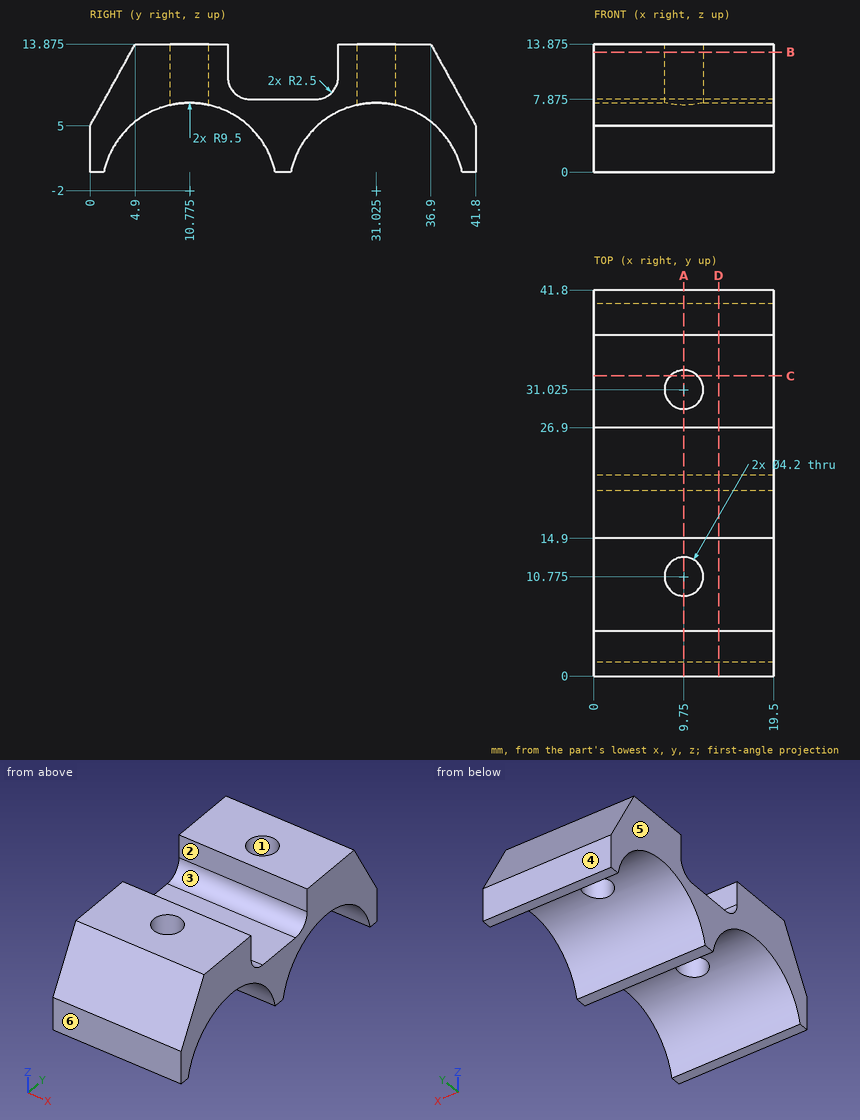
Study the drawing (mm; zero at the part's minimum x, y, z) and answer. A direction names the side the tool comes from. Give positions to 0.01 mm unless a question says otherwise; leave off trailing zeros. Order: outer loops, then holes, each group sorted by start corner. A loop starts at its lowest first (then second) coordinate and runs counter-clockwise, first axis right, second up. Notation, with made-up numbers: (6, -13.75) -> (58, -13.75) arc R15 cw to (58, -7.75) -> close; hole circle Ø8 at (13.5, 13). An arc over 180 degrees is marked (long way). Put each result on its own line as item: value.
Item 1: A cutting plane is placed at B-B on z = 13. Give the vertices of the cut face in (x, y) (3 decimals), plus the area to 3 significant figures.
Established:
outline: (0, 4.417) -> (19.5, 4.417) -> (19.5, 14.9) -> (0, 14.9) -> close; (0, 26.9) -> (19.5, 26.9) -> (19.5, 37.383) -> (0, 37.383) -> close; hole circle Ø4.2 at (9.75, 10.775); hole circle Ø4.2 at (9.75, 31.025)
area: 381 mm^2
Item 2: Straight lines are drawn through the part: line 1 (Y direction, x = 11.75, z = 6.75); line 2 (Y direction, x = 9.75, z = 11) (3 decimals); line 3 (Y direction, x = 9.75, z = 12.75) (3 decimals). For each, find the intervals that lie inside material, in ascending order.
Established:
line 1: y = 0.97 to 7.08, 14.47 to 27.33, 34.72 to 40.83
line 2: y = 3.313 to 8.675, 12.875 to 14.9, 26.9 to 28.925, 33.125 to 38.487
line 3: y = 4.279 to 8.675, 12.875 to 14.9, 26.9 to 28.925, 33.125 to 37.521
Item 3: A cutting plane is placed at C-C on y = 32.5. Give the vertices of the cut face in (x, z) (3 decimals).
Established:
outline: (0, 7.385) -> (8.255, 7.385) -> (8.255, 13.875) -> (0, 13.875) -> close; (11.245, 7.385) -> (19.5, 7.385) -> (19.5, 13.875) -> (11.245, 13.875) -> close
Item 4: Given P1, Ø1, axis at x = 9.5, z = 6, coming from the +Y side; P2, Ø1, axis at x = 8, z = 11.5, coming from the +Y side; P3, Ø2, axis at x = 15, y = 37, coming from the -Z side, each flat-ended and moving along its own axis, determine where each tip first touches the part or whether it passes through.
Established:
P1: stops at y = 41.52
P2: stops at y = 38.49
P3: stops at z = 4.45
Item 5: A cutting plane is placed at A-A on x = 9.75. Give the vertices of the cut face in (y, z) (3 decimals).
Established:
outline: (0, 0) -> (1.488, 0) arc R9.5 cw to (8.675, 7.265) -> (8.675, 13.875) -> (4.9, 13.875) -> (0, 5) -> close; (12.875, 7.265) arc R9.5 cw to (20.062, 0) -> (21.738, 0) arc R9.5 cw to (28.925, 7.265) -> (28.925, 13.875) -> (26.9, 13.875) -> (26.9, 10.375) arc R2.5 cw to (24.4, 7.875) -> (17.4, 7.875) arc R2.5 cw to (14.9, 10.375) -> (14.9, 13.875) -> (12.875, 13.875) -> close; (33.125, 7.265) arc R9.5 cw to (40.312, 0) -> (41.8, 0) -> (41.8, 5) -> (36.9, 13.875) -> (33.125, 13.875) -> close
Item 6: For a pull along Y with two mould halves and no side action, classify the marked faces 3, 4, 5 and 6 as released by +Y, released by -Y, zero draft, split by the parting line, or undercut.
Established:
face 3: undercut
face 4: released by +Y
face 5: zero draft
face 6: released by -Y
Item 7: A cutting plane is placed at D-D on x = 13.5. Give the vertices of the cut face in (y, z) (3 decimals), plus the area to 3 significant figures.
Established:
outline: (0, 0) -> (1.488, 0) arc R9.5 cw to (20.062, 0) -> (21.738, 0) arc R9.5 cw to (40.312, 0) -> (41.8, 0) -> (41.8, 5) -> (36.9, 13.875) -> (26.9, 13.875) -> (26.9, 10.375) arc R2.5 cw to (24.4, 7.875) -> (17.4, 7.875) arc R2.5 cw to (14.9, 10.375) -> (14.9, 13.875) -> (4.9, 13.875) -> (0, 5) -> close
area: 259 mm^2
Item 8: For the marked faces 1 and 2, determine the directions among +Z, -Z, +X, -X, +Y, -Y from which every point of the face is accessible in a straight line to the end or side of a thin tool.
Established:
face 1: +Z, -Z
face 2: +Z, +X, -X
